Verification items for the finished model (mm, model axes). Face numbers are marked on the shaded views. A direction names the side the tool comes from. Round coordinates to 2 decimals unless told otherwise and drop trailing zeros. Loops run counter-clockwise (first coordinate to the right, second up) from the corner with the lowest first, then second, coordinate; pieces in that order, holes last. Notation, with made-up numbers: M 10.25,25 L 46.25,25 A38 ccw 46.25,63 Z; hole C 1.5,68 d6. An arc over 180 degrees is marked long. Answer as CSV lines item,"result".
```python
from build123d import *

# Parameters (mm, degrees)
ESQUISSE1_R           = 23.25
ESQUISSE1_R_2         = 20.75
MAIN_DEPTH            = 8
ESQUISSE2_R           = 20.75
CENTRALPART_DEPTH     = 2
HEXAGONAL_DEPTH       = 6
ESQUISSE5_R           = 4
CENTRALHOLE_DEPTH     = 6
SKETCH1_R             = 1.25
FIXTOPHOLE_DEPTH      = 3.25
FIXTOPHOLE_DEPTH_BACK = 22
SKETCH2_R             = 5
CUT_EXTRUDE2_DEPTH    = 3.250000111
SKETCH3_R             = 1.25
HUBFIXHOLE_DEPTH      = 9.0000001
CIRPATTERN1_COUNT     = 8


with BuildPart() as part:
    # Esquisse1 → Main (new body, symmetric)
    with BuildSketch(Plane.XY):
        Circle(ESQUISSE1_R)
        Circle(ESQUISSE1_R_2, mode=Mode.SUBTRACT)
    extrude(amount=MAIN_DEPTH, both=True)

    # Esquisse2 → CentralPart (add, symmetric)
    with BuildSketch(Plane.XY):
        Circle(ESQUISSE2_R)
    extrude(amount=CENTRALPART_DEPTH, both=True)

    # Esquisse3 → Hexagonal (add)
    with BuildSketch(Plane.XY):
        Polygon((-3.464101615, 6), (-6.92820323, 0), (-3.464101615, -6), (3.464101615, -6), (6.92820323, 0), (3.464101615, 6), align=None)
    extrude(amount=HEXAGONAL_DEPTH)

    # Esquisse5 → CentralHole (cut, symmetric)
    with BuildSketch(Plane.XY):
        Circle(ESQUISSE5_R)
    extrude(amount=CENTRALHOLE_DEPTH, both=True, mode=Mode.SUBTRACT)

    # Sketch1 → FixTopHole (cut, two sides)
    with BuildSketch(Plane(origin=(0, 21, 0), x_dir=(1, 0, 0), z_dir=(0, 1, 0))) as fixtophole_sk:
        Circle(SKETCH1_R)
    extrude(amount=FIXTOPHOLE_DEPTH, mode=Mode.SUBTRACT)
    extrude(fixtophole_sk.sketch, amount=-FIXTOPHOLE_DEPTH_BACK, mode=Mode.SUBTRACT)

    # Sketch2 → Cut-Extrude2 (cut, through all)
    with BuildSketch(Plane(origin=(0, 21, 0), x_dir=(1, 0, 0), z_dir=(0, 1, 0))):
        Circle(SKETCH2_R)
    extrude(amount=CUT_EXTRUDE2_DEPTH, mode=Mode.SUBTRACT)

    # Sketch3 → HubFixHole (cut, symmetric)
    with BuildSketch(Plane.XY):
        with Locations((-6.314276634, 15.244012286)):
            Circle(SKETCH3_R)
    hubfixhole = extrude(amount=HUBFIXHOLE_DEPTH, both=True, mode=Mode.SUBTRACT)

    # CirPattern1: HubFixHole ×8 about axis
    cirpattern1_axis = Axis((0, 0, 0), (0, 0, 1))
    for i in range(1, CIRPATTERN1_COUNT):
        add(hubfixhole.rotate(cirpattern1_axis, i * 360 / CIRPATTERN1_COUNT), mode=Mode.SUBTRACT)


solid = part.part
```
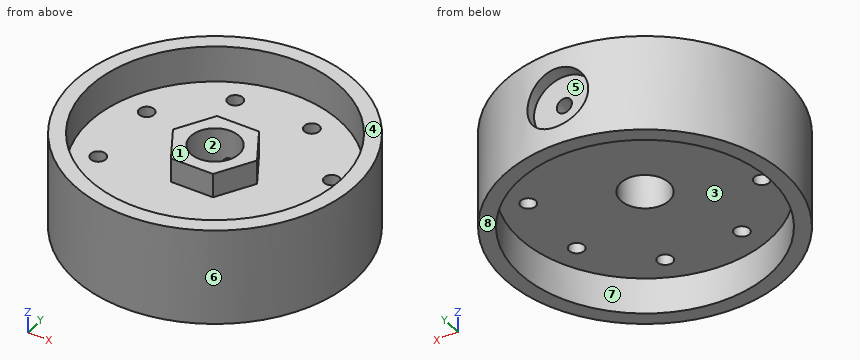
1) Set-up check for the marked faces 1, 2, 3, 4 and 5: record each of +Z, -Z, +X, -X, +Y, -Y from which the full face is reachable in a straight line by a thin tool's end or side.
Here are the results:
face 1,"+Z"
face 2,"+Z, -Z"
face 3,"-Z"
face 4,"+Z, +X, -X, +Y, -Y"
face 5,"+Y"
2) Section check A-A (x = 0). Record the cut outline in (y, z), plus the area to 3 significant figures.
Here are the results:
outline,"M -23.25,-8 L -20.75,-8 L -20.75,-2 L -4,-2 L -4,6 L -6,6 L -6,2 L -20.75,2 L -20.75,8 L -23.25,8 Z; M 4,-2 L 20.75,-2 L 20.75,-8 L 23.25,-8 L 23.25,-5 L 21,-5 L 21,-1.25 L 4,-1.25 Z; M 4,1.25 L 21,1.25 L 21,5 L 23.25,5 L 23.25,8 L 20.75,8 L 20.75,2 L 6,2 L 6,6 L 4,6 Z"
area,"165 mm^2"
3) Section check C-C (z = 3.5). Record the cut outline in (x, y).
Here are the results:
outline,"M -6.93,0 L -3.46,-6 L 3.46,-6 L 6.93,0 L 3.46,6 L -3.46,6 Z; M -3.57,21 L -3.57,22.97 A23.25 ccw long 3.57,22.97 L 3.57,21 Z; hole C 0,0 d41.5; hole C 0,0 d8"
4) Section check B-B (y = 1). Record the cut outline in (x, z).
Here are the results:
outline,"M -23.23,-8 L -20.73,-8 L -20.73,-2 L -3.87,-2 L -3.87,6 L -6.35,6 L -6.35,2 L -20.73,2 L -20.73,8 L -23.23,8 Z; M 3.87,-2 L 20.73,-2 L 20.73,-8 L 23.23,-8 L 23.23,8 L 20.73,8 L 20.73,2 L 6.35,2 L 6.35,6 L 3.87,6 Z"
5) Section check D-D (z = 0). State how many separate pieces and enclosed holes the cut face has, plus the area to 3 significant figures.
Here are the results:
separate pieces,"1"
enclosed holes,"8"
area,"1,550 mm^2"
6) Draft check along X on the marked faces 6, 7 and 8. Enter one of: +X half, -X half, draft (parallel to the pull), parting line (faces both ways), or undercut.
Here are the results:
face 6,"parting line"
face 7,"undercut"
face 8,"draft"
7) Go/stop test with flat-tipped pins: pin 1 (5 mm diameter, centred on x = -16.5, y = 3.5, fed in from -Z); pin 2 (5 mm diameter, centred on x = -7.5, z = -2.5, fed in from -Y); pin 3 (13 mm diameter, centred on x = -1, y = -2.5, fed in from +Z). Record where each tip stops, or that it passes through.
Here are the results:
pin 1,"stops at z = -2"
pin 2,"stops at y = -22.71"
pin 3,"stops at z = 6"
8) Material ranges on probe 1 along X at (y, z) = (-15, 1.5); probe 2 along Z at (x, y) = (0, 21.7); probe 3 along Z at (x, y) = (15.5, -11), recorded low to high.
Here are the results:
probe 1,"x = -17.76 to -7.54, -5.09 to 5.09, 7.54 to 17.76"
probe 2,"z = -8 to -5, 5 to 8"
probe 3,"z = -2 to 2"
